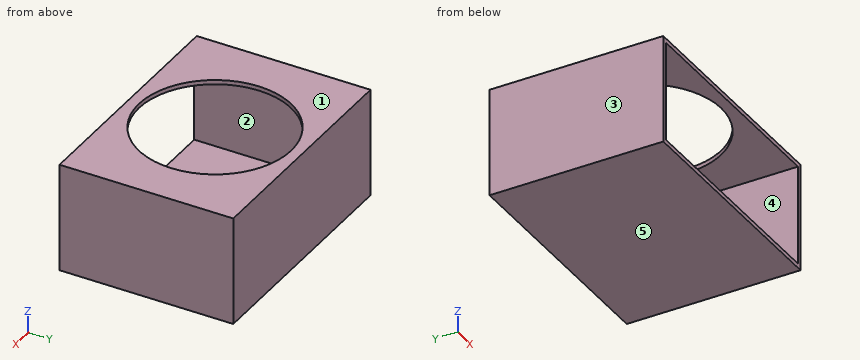
from build123d import *

# Parameters (mm, degrees)
SKETCH_1_W          = 110
SKETCH_1_H          = 50
EXTRUDE_1_DEPTH     = 80
SHELL_1_T           = -2
SKETCH_2_R          = 35
CUT_EXTRUDE_1_DEPTH = 2


with BuildPart() as part:
    # 草图1 → 凸台-拉伸1 (new body)
    with BuildSketch(Plane(origin=(0, 0, 0), x_dir=(1, 0, 0), z_dir=(0, 1, 0))):
        Rectangle(SKETCH_1_W, SKETCH_1_H)
    extrude(amount=EXTRUDE_1_DEPTH)

    # 抽壳1
    shell_1_openings = [part.faces().sort_by_distance(p)[0] for p in [
        (0, 0, 0),
    ]]
    offset(amount=SHELL_1_T, openings=shell_1_openings, kind=Kind.INTERSECTION)

    # 草图2 → 切除-拉伸1 (cut)
    with BuildSketch(Plane.XY.offset(25)):
        with Locations((0, 40)):
            Circle(SKETCH_2_R)
    extrude(amount=-CUT_EXTRUDE_1_DEPTH, mode=Mode.SUBTRACT)


solid = part.part
Input: part model. Units: mm. Frame: model coordinates. Face numbers are marked on the shaded views. A direction names the side the tool comes from. Give positions to 0.01 mm unless a question says otherwise; leave off trailing zeros. Write each loop counter-clockwise with the first axis right and the second up, starting at its lowest first coordinate (ties: lowest second). Pieces come first, ordered by that corner, then holes.
Q1. Material intervals for probe 1 along Y at (x, z) = (0, 24); probe 2 along X at (y, z) = (60.5, 13); probe 3 along Z at (x, y) = (-51, 41.5), sorted ascending.
Q2. Section A-A, the plane x = 0. Output: boundary loops of the cut face in (y, z), plus the area to 3 significant figures.
Q3. Section C-C, the plane x = 48.5. Output: boundary loops of the cut face in (y, z).
Q4. Pull-direction query (Z, two-part tool) for the marked faces 1, 2 and 3; classes: pulls with the +Z half, pulls with the -Z half, needs draft (parallel to the pull), parting line crosses it, or undercut.
Q5. Section D-D, the plane z = 2. Output: boundary loops of the cut face in (x, y), plus the area to 3 significant figures.
Q6. First-contact query: P1, Ø2, axis at x = -7, z = -18, coming from the -Y side. Flat tip, straight axial feed; report the tip coordinate or a pass-through.
Q7. Section B-B, the plane y = 40. Output: boundary loops of the cut face in (x, z).
Q8. Set-up query: the marked faces 4 and 5. Return all of +Z, -Z, +X, -X, +Y, -Y with unobstructed straight access to the full face (end or side cutting, diameter ignored); none if empty.
Filled in:
1. probe 1: y = 0 to 5, 75 to 80
1. probe 2: x = -55 to -53, 53 to 55
1. probe 3: z = -25 to -23, 23 to 25
2. outline: (0, -25) - (80, -25) - (80, 25) - (75, 25) - (75, 23) - (78, 23) - (78, -23) - (0, -23) - close; (0, 23) - (5, 23) - (5, 25) - (0, 25) - close
2. area: 272 mm2
3. outline: (0, -25) - (80, -25) - (80, 25) - (0, 25) - (0, 23) - (78, 23) - (78, -23) - (0, -23) - close
4. face 1: pulls with the +Z half
4. face 2: undercut
4. face 3: needs draft
5. outline: (-55, 0) - (-53, 0) - (-53, 78) - (53, 78) - (53, 0) - (55, 0) - (55, 80) - (-55, 80) - close
5. area: 532 mm2
6. P1: stops at y = 78
7. outline: (-55, -25) - (55, -25) - (55, 25) - (35, 25) - (35, 23) - (53, 23) - (53, -23) - (-53, -23) - (-53, 23) - (-35, 23) - (-35, 25) - (-55, 25) - close
8. face 4: -Y
8. face 5: -Z, +X, -X, +Y, -Y
